Design review of the part built by this model. Coordinates are the model's own, in mm. Face numbers are marked on the shaded views. A direction names the side the tool comes from. Give positions to 0.01 mm unless a question says otherwise; leave off trailing zeros. Write each loop counter-clockwise with the first axis right and the second up, starting at its lowest first coordinate (ties: lowest second). Pieces come first, ordered by that corner, then holes. Notation, with made-up numbers: M 22,77.25 L 36,77.25 A16 cw 36,94.25 Z; hole C 54,23 d10. An arc over 180 degrees is marked long. One line per item, written item: value. Start each with the question number.
Autodesk Fusion 360 part; units mm, degrees
sketch "Sketch1" plane through (0, 0, 0) normal (0, 1, 0) x (1, 0, 0)
  arc A0 (31.1232, 52.6914) -> (20.5609, 48.637) centre (27.8693, 45.3831) ccw
  line L0 (31.1232, 52.6914) -> (40.2587, 48.6241)
  arc A1 (28.2837, -48.2895) -> (32.9132, -32.6608) centre (28.2837, -39.7895) ccw
  line L1 (28.2837, -48.2895) -> (-42.2163, -48.2895)
  arc A2 (-4.6567, -8.0029) -> (-2.8122, -14.2299) centre (-0.089, -10.0365) ccw
  line L2 (22.8004, 52.0184) -> (38.6317, 44.9699)
  line L3 (-46.7163, -32.2895) -> (-50.7163, -32.2895)
  line L4 (35.3386, -39.0053) -> (-23.3345, -39.0053) construction
  arc A3 (28.2837, -44.2895) -> (30.7346, -36.0155) centre (28.2837, -39.7895) ccw
  line L5 (40.2587, 48.6241) -> (38.6317, 44.9699)
  line L6 (30.7346, -36.0155) -> (-2.8122, -14.2299)
  line L7 (-50.7163, -39.7895) -> (-50.7163, -32.2895)
  line L8 (32.9132, -32.6608) -> (-0.6336, -10.8752)
  arc A4 (-46.7163, -39.7895) -> (-42.2163, -44.2895) centre (-42.2163, -39.7895) ccw
  arc A5 (-50.7163, -39.7895) -> (-42.2163, -48.2895) centre (-42.2163, -39.7895) ccw
  line L9 (-4.6567, -8.0029) -> (20.5609, 48.637)
  line L10 (28.2837, -44.2895) -> (-42.2163, -44.2895)
  line L11 (-46.7163, -39.7895) -> (-46.7163, -32.2895)
  arc A6 (22.8004, 52.0184) -> (27.1963, 53.7059) centre (27.8693, 45.3831) ccw
  arc A7 (-1.0025, -9.6298) -> (-0.6336, -10.8752) centre (-0.089, -10.0365) ccw
  line L12 (-1.0025, -9.6298) -> (27.1963, 53.7059)
  point P0 (35.3386, -39.0053)
  point P1 (-46.7163, -44.2895)
  point P2 (23.8148, 55.9453)
  dimension "d1" = 33
  dimension "d2" = 66
  dimension "d3" = 4.5
  dimension "d4" = 5
  dimension "d5" = 12
  dimension "d6" = 18
  dimension "d10" = 75
  dimension "d11" = 70
  dimension "d12" = 40
  dimension "d13" = 8
  dimension "d14" = 4.5
extrude "Extrude1" add sketch "Sketch1" along normal blind 75 contours A0 L2 L9 A6 L12 | A1 L1 A2 L3 A3 L6 L7 L8 A4 A5 L9 L10 L11 A6 A7 L12
sketch "Sketch2" plane through (-0.9127, 0, -0.4064) normal (-0.9135, 0, -0.4067) x (-0.4067, 0, 0.9135)
  line L0 (-52.795, 0) -> (9.205, 0)
  line L1 (9.205, 0) -> (9.205, 75)
  line L2 (9.205, 75) -> (-52.795, 75)
  line L3 (-52.795, 75) -> (-52.795, 0)
  circle A0 centre (-42.795, 37.5) radius 4
  circle A1 centre (-12.795, 37.5) radius 4
  line L4 (-31.6238, 0) -> (-31.6238, 75)
  line L5 (9.205, 37.5) -> (-64.6996, 37.5)
  dimension "d17" = 8
  dimension "d18" = 8
  dimension "d23" = 10
  dimension "d24" = 30
extrude "Extrude2" cut sketch "Sketch2" along normal blind 18 and the other way blind 25 contours A0 L5 | A0 L5 | A1 L5 | A1 L5
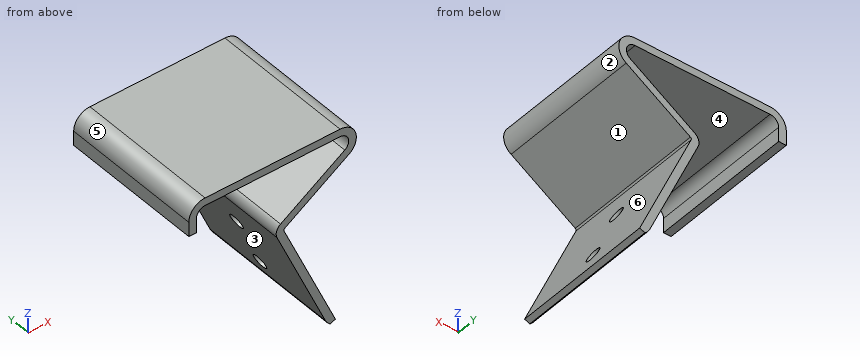
Q1. For P1, Ø6, axis at x = 23, y = 42, coming from the -Z side; P2, Ø3, axis at x = -33, y = 42.5, coming from the -Z side; P3, Ø21, axis at x = -9.5, y = 27, coming from the -Z side, all flat-tipped, find the tip position at first contact; note any pin that passes through.
Q2. The part is to be moulded in two halves that separate along Z. For the marked faces 1, 2 and 3, say which applies: pulls with the +Z half, pulls with the -Z half, needs draft (parallel to the pull), parting line crosses it, or undercut.
Q3. Wall thickness on line 1 (Z direction, x = 2.5, y = 44); line 2 (Z direction, x = 12.5, y = 19); line 3 (Z direction, x = -5.5, y = 69): over which ranges is each line inside the solid? List them lowest first. Write a range as from..to.
Q4. Machinability: for the marked faces 4, 5 and 6, which of the approach directions +Z, -Z, +X, -X, +Y, -Y give a long, thin tool a straight path to every point of the face, cutting with its end or side? Answer none if there is none.
Q5. Take a section at D-D, the plane x = -13. Give the boundary of the cut face in (y, z), then the cut area to 3 significant figures.
Q6. Take a section at B-B, the plane y = 39. Give the boundary of the cut face in (x, z), then the cut area to 3 significant figures.
Q7. Take a section at C-C, the plane y = 26. Give the boundary of the cut face in (x, z).
Q8. Take a section at A-A, the plane x = 13. Give the boundary of the cut face in (y, z), then the cut area to 3 significant figures.
Results list:
1. P1: stops at z = -51.86
1. P2: stops at z = 44.29
1. P3: stops at z = -4.7
2. face 1: undercut
2. face 2: parting line crosses it
2. face 3: pulls with the -Z half
3. line 1: z = -8.07..1.76, 12.91..17.68, 44.29..48.29
3. line 2: z = -30.53..-20.7, 19.4..24.17, 44.29..48.29
3. line 3: z = 44.29..48.29
4. face 4: +Y, -Y
4. face 5: +Z, -X, +Y, -Y
4. face 6: +X, +Y, -Y
5. outline: M 0,44.29 L 75,44.29 L 75,48.29 L 0,48.29 Z
5. area: 300 mm^2
6. outline: M -50.72,32.29 L -46.72,32.29 L -46.72,39.79 A4.5 cw -42.22,44.29 L 28.28,44.29 A4.5 cw 30.73,36.02 L -2.81,14.23 A5 ccw -4.66,8 L 2.78,-8.71 L 6.44,-7.08 L -1,9.63 A1 cw -0.63,10.88 L 32.91,32.66 A8.5 ccw 28.28,48.29 L -42.22,48.29 A8.5 ccw -50.72,39.79 Z; M 5.8,-15.48 L 14.99,-36.11 L 18.64,-34.49 L 9.45,-13.86 Z; M 18,-42.89 L 20.56,-48.64 A8 ccw 23.17,-51.86 L 25.84,-50.66 L 21.66,-41.26 Z
6. area: 800 mm^2
7. outline: M -50.72,32.29 L -46.72,32.29 L -46.72,39.79 A4.5 cw -42.22,44.29 L 28.28,44.29 A4.5 cw 30.73,36.02 L -2.81,14.23 A5 ccw -4.66,8 L 20.56,-48.64 A8 ccw 23.17,-51.86 L 25.84,-50.66 L -1,9.63 A1 cw -0.63,10.88 L 32.91,32.66 A8.5 ccw 28.28,48.29 L -42.22,48.29 A8.5 ccw -50.72,39.79 Z
8. outline: M 0,-31.65 L 75,-31.65 L 75,-21.82 L 0,-21.82 Z; M 0,19.73 L 75,19.73 L 75,24.5 L 0,24.5 Z; M 0,44.29 L 75,44.29 L 75,48.29 L 0,48.29 Z
8. area: 1,400 mm^2
